Model file for the job. Use its own axes, mm. Face numbers are marked on the shaded views. Coordinates: 2 decimals unless noted, no trailing zeros. Order: outer loops, then holes, each group sorted by start corner. A loop starts at its lowest first (then second) coordinate and runs counter-clockwise, first axis right, second up. Notation, with made-up numbers: (-11.5, -16.5) -> (24.5, -16.5) arc R29 ccw to (24.5, 14.5) -> close; hole circle Ø3 at (81.5, 69.5). An arc over 180 degrees is marked (long way). Use CSV: the item, a comma, the result in double quotes. Start each with the question number.
(1) Pin check, flat tips, straight feed: pin 1 Ø1.4 at (y, z) = (2, -55) entering from +X; pin 2 Ø10 at (x, z) = (8.5, -35) entering from +Y; pin 3 Ø3 at (x, y) = (7, 15) entering from -Z. Stop position of each tip, or through.
(2) Probe L1, parallel to Y at x = 0, z = -40.25; L2, parallel to X at y = 15, z = 2; L3, parallel to Z at x = 1, y = -10. List the from-to ranges inside material, lowest first.
(3) Cut at A-A on z = -2.5. Write the cut outline in (x, y).
(4) Cut at C-C on z = -16.5. Write the cut outline in (x, y).
(5) Cut at B-B on y = -14.5. Give the number of separate pieces and of enclosed holes in the cut face, plus the area to 3 significant figures.
(6) Pull direction X, two halves, no side cores. Call the marked faces 1, 2 and 3: pulls with the +X half, pulls with the -X half, needs draft (parallel to the pull), parting line crosses it, or undercut.
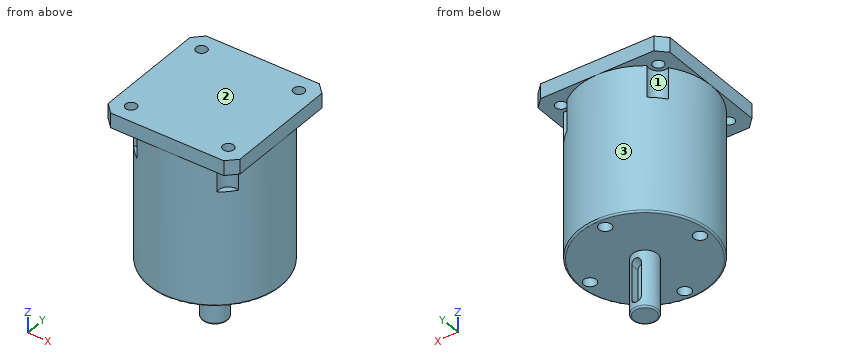
```python
from build123d import *

# Parameters (mm, degrees)
BOSS_EXTRUDE1_DEPTH = 4.7
SKETCH2_R           = 21
BOSS_EXTRUDE2_DEPTH = 51
SKETCH3_R           = 4
BOSS_EXTRUDE3_DEPTH = 18
SKETCH5_R           = 1.75
CUT_EXTRUDE1_DEPTH  = 10
SKETCH6_R           = 3
CUT_EXTRUDE2_DEPTH  = 10
CUT_EXTRUDE3_DEPTH  = 3
FILLET1_R           = 0.5
SKETCH8_R           = 2
CUT_EXTRUDE4_DEPTH  = 10


with BuildPart() as part:
    # Sketch1 → Boss-Extrude1 (new body)
    with BuildSketch(Plane.XY):
        Polygon((-21, 18), (-18, 21), (18, 21), (21, 18), (21, -18), (18, -21), (-18, -21), (-21, -18), align=None)
    extrude(amount=BOSS_EXTRUDE1_DEPTH)

    # Sketch2 → Boss-Extrude2 (add)
    with BuildSketch(Plane.XY.offset(4.7)):
        Circle(SKETCH2_R)
    extrude(amount=-BOSS_EXTRUDE2_DEPTH)

    # Sketch3 → Boss-Extrude3 (add)
    with BuildSketch(Plane(origin=(0, 0, -46.3), x_dir=(-1, 0, 0), z_dir=(0, 0, -1))):
        Circle(SKETCH3_R)
    extrude(amount=BOSS_EXTRUDE3_DEPTH)

    # Sketch5 → Cut-Extrude1 (cut)
    with BuildSketch(Plane.XY.offset(4.7)):
        with Locations((-15.5, 15.5)):
            Circle(SKETCH5_R)
        with Locations((15.5, 15.5)):
            Circle(SKETCH5_R)
        with Locations((-15.5, -15.5)):
            Circle(SKETCH5_R)
        with Locations((15.5, -15.5)):
            Circle(SKETCH5_R)
    extrude(amount=-CUT_EXTRUDE1_DEPTH, mode=Mode.SUBTRACT)

    # Sketch6 → Cut-Extrude2 (cut)
    with BuildSketch(Plane(origin=(0, 0, 0), x_dir=(-1, 0, 0), z_dir=(0, 0, -1))):
        with Locations((-15.5, 15.5)):
            Circle(SKETCH6_R)
        with Locations((-15.5, -15.5)):
            Circle(SKETCH6_R)
        with Locations((15.5, -15.5)):
            Circle(SKETCH6_R)
        with Locations((15.5, 15.5)):
            Circle(SKETCH6_R)
    extrude(amount=CUT_EXTRUDE2_DEPTH, mode=Mode.SUBTRACT)

    # Sketch7 → Cut-Extrude3 (cut)
    with BuildSketch(Plane(origin=(0, 4, 0), x_dir=(1, 0, 0), z_dir=(0, 1, 0))):
        with BuildLine():
            Line((1.5, 60.8), (1.5, 49.8))
            ThreePointArc((1.5, 49.8), (0, 48.3), (-1.5, 49.8))
            Line((-1.5, 49.8), (-1.5, 60.8))
            ThreePointArc((-1.5, 60.8), (0, 62.3), (1.5, 60.8))
        make_face()
    extrude(amount=-CUT_EXTRUDE3_DEPTH, mode=Mode.SUBTRACT)

    # Fillet1
    fillet1_edges = [part.edges().sort_by_distance(p)[0] for p in [
        (-21, 0, -46.3),
        (4, 0, -64.3),
    ]]
    fillet(fillet1_edges, radius=FILLET1_R)

    # Sketch8 → Cut-Extrude4 (cut)
    with BuildSketch(Plane(origin=(0, 0, -46.3), x_dir=(-1, 0, 0), z_dir=(0, 0, -1))):
        with Locations((0, 17.5)):
            Circle(SKETCH8_R)
        with Locations((-17.5, 0)):
            Circle(SKETCH8_R)
        with Locations((0, -17.5)):
            Circle(SKETCH8_R)
        with Locations((17.5, 0)):
            Circle(SKETCH8_R)
    extrude(amount=-CUT_EXTRUDE4_DEPTH, mode=Mode.SUBTRACT)


solid = part.part
```
Outcome:
1,pin 1,"x = 3.78"
1,pin 2,"y = 20.71"
1,pin 3,"z = -46.3"
2,L1,"-21 to -19.5, -15.5 to 15.5, 19.5 to 21"
2,L2,"-21 to -17.18, -13.82 to 13.82, 17.18 to 21"
2,L3,"-46.3 to 4.7"
3,outline,"(-16.69, -12.75) arc R3 cw to (-12.75, -16.69) arc R21 ccw to (12.75, -16.69) arc R3 cw to (16.69, -12.75) arc R21 ccw to (16.69, 12.75) arc R3 cw to (12.75, 16.69) arc R21 ccw to (-12.75, 16.69) arc R3 cw to (-16.69, 12.75) arc R21 ccw to start"
4,outline,"circle Ø42 at (0, 0)"
5,separate pieces,"3"
5,enclosed holes,"0"
5,area,"1,530 mm2"
6,face 1,"undercut"
6,face 2,"needs draft"
6,face 3,"parting line crosses it"
